Check sheet for the modelled part. Datum: model origin and axes. Units: mm. Round coordinates to 2 decimals unless told otherwise and drop trailing zeros. Order: outer loops, then holes, each group sorted by start corner. A loop starts at its lowest first (then second) coordinate and runs counter-clockwise, first axis right, second up.
(1) Sectioned sample at A-A, the plane z = 0.75. Count the separate pieces of the cut face and the enclosed holes in it, and give its area (3 significant figures).
(2) Sectioned sample at B-B, the plane y = 12. Enter the section's corners in (x, z).
(3) Sectioned sample at C-C, the plane x = 52. Enter the section's corners in (y, z), and give its area (4 significant figures).
(4) Thickness scan on probe 1 along X at (y, z) = (15, 0.5); probe 2 along Y at (x, z) = (62, 0.85). Record the ranges inside material, lowest first.
(5) Depth check by flat-ended pin: pin 1 (0.8 mm diameter, centred on x = 45.5, z = 0.5, fed in from +Y); pin 2 (0.8 mm diameter, centred on y = -15, z = 1, fed in from -X). Enter the tip coordinate at first touch or a pass-through.
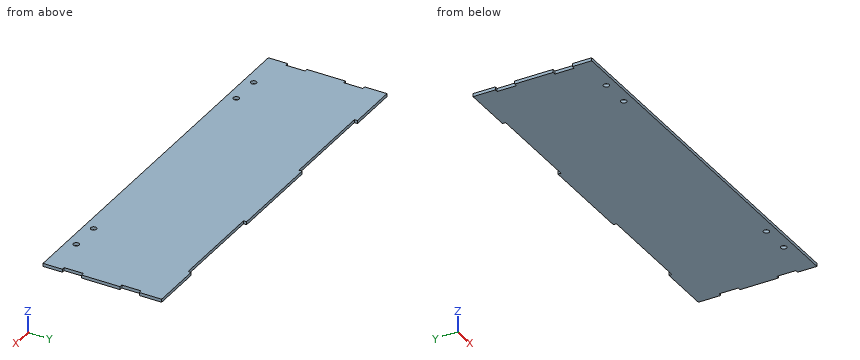
```python
from build123d import *

# Parameters (mm, degrees)
F0_W     = 1.5875
F0_H     = 20
F0_H_2   = 10
F0_W_2   = 50
F0_H_3   = 1.5875
F0_W_3   = 200
F0_R     = 1.4732
F1_DEPTH = 1.5875


# Not quite as in the source:
# - a length typed as a fraction of an inch, garbled in the dataset ("3 / 203.2 mm" for 3/8 in), is restored


with BuildPart() as f1:
    # F0 (on Top) → F1 (new body)
    with BuildSketch(Plane.XY):
        with Locations((100.8545614919, -1.1143145161)):
            Rectangle(F0_W, F0_H)
        with Locations((-100.7329385081, -1.1143145161)):
            Rectangle(F0_W, F0_H)
        with Locations((-100.7329385081, -26.1143145161)):
            Rectangle(F0_W, F0_H_2)
        with Locations((100.8545614919, 23.8856854839)):
            Rectangle(F0_W, F0_H_2)
        with Locations((-100.7329385081, 23.8856854839)):
            Rectangle(F0_W, F0_H_2)
        with Locations((100.8545614919, -26.1143145161)):
            Rectangle(F0_W, F0_H_2)
        Polygon((75.0608114919, 28.8856854839), (100.0608114919, 28.8856854839), (101.6483114919, 28.8856854839), (101.6483114919, 30.4731854839), (75.0608114919, 30.4731854839), align=None)
        with Locations((0.0608114919, 29.6794354839)):
            Rectangle(F0_W_2, F0_H_3)
        Polygon((-101.5266885081, 28.8856854839), (-99.9391885081, 28.8856854839), (-74.9391885081, 28.8856854839), (-74.9391885081, 30.4731854839), (-101.5266885081, 30.4731854839), align=None)
        Polygon((100.0608114919, 8.8856854839), (100.0608114919, 18.8856854839), (-99.9391885081, 18.8856854839), (-99.9391885081, 8.8856854839), (-99.9391885081, -11.1143145161), (-99.9391885081, -21.1143145161), (100.0608114919, -21.1143145161), (100.0608114919, -11.1143145161), align=None)
        with Locations((0.0608114919, -26.1143145161)):
            Rectangle(F0_W_3, F0_H_2)
        with Locations((-79.9391885081, -26.3018145161)):
            Circle(F0_R, mode=Mode.SUBTRACT)
        with Locations((-64.2419885081, -26.3018145161)):
            Circle(F0_R, mode=Mode.SUBTRACT)
        with Locations((64.3636114919, -26.3018145161)):
            Circle(F0_R, mode=Mode.SUBTRACT)
        with Locations((80.0608114919, -26.3018145161)):
            Circle(F0_R, mode=Mode.SUBTRACT)
        Polygon((-99.9391885081, 18.8856854839), (100.0608114919, 18.8856854839), (100.0608114919, 28.8856854839), (75.0608114919, 28.8856854839), (25.0608114919, 28.8856854839), (-24.9391885081, 28.8856854839), (-74.9391885081, 28.8856854839), (-99.9391885081, 28.8856854839), align=None)
    extrude(amount=F1_DEPTH)


solid = f1.part
```
Derived:
1. separate pieces: 1
1. enclosed holes: 4
1. area: 12,300 mm2
2. outline: (-99.94, 0) - (100.06, 0) - (100.06, 1.59) - (-99.94, 1.59) - close
3. outline: (-31.11, 0) - (28.89, 0) - (28.89, 1.59) - (-31.11, 1.59) - close
3. area: 95.25 mm2
4. probe 1: x = -99.94 to 100.06
4. probe 2: y = -31.11 to 28.89
5. pin 1: stops at y = 28.89
5. pin 2: stops at x = -99.94
